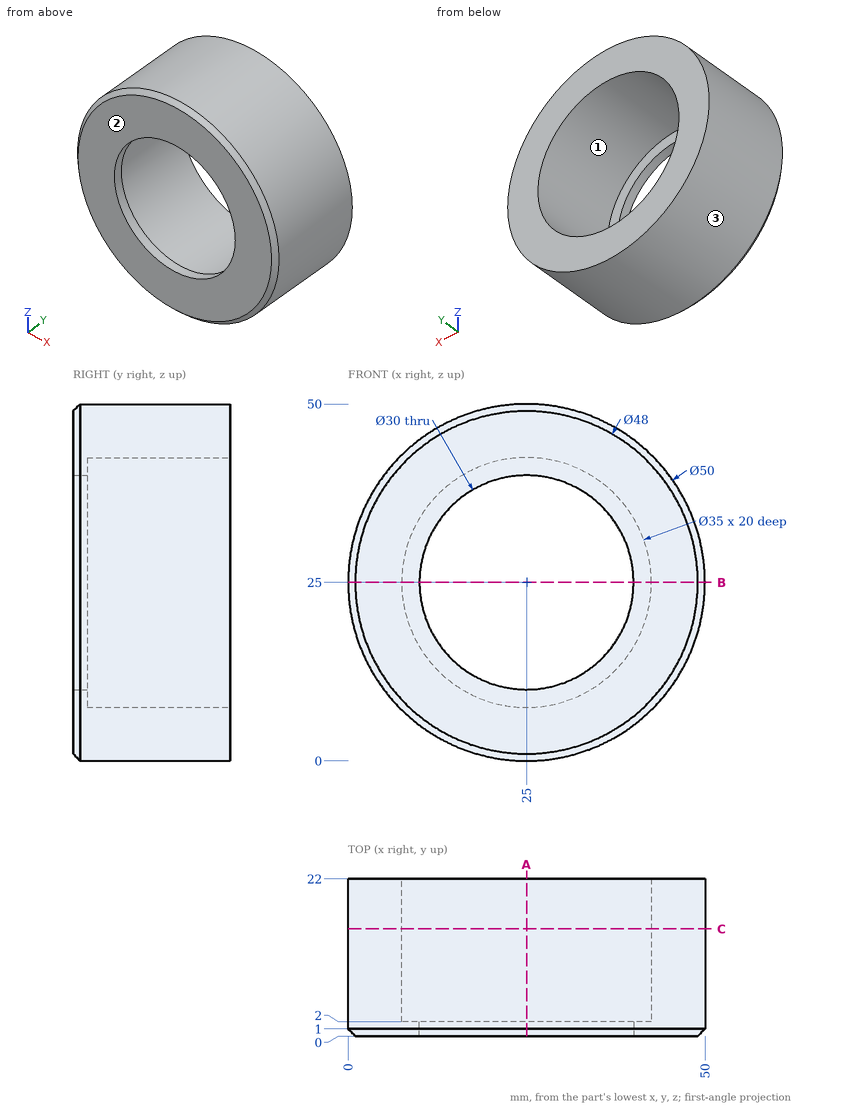
Study the drawing (mm; zero at the part's minimum x, y, z) and answer. Round coordinates to 2 decimals unless told otherwise and drop trailing zeros. Loops run counter-clockwise (first coordinate to the right, second up) from the corner with the lowest first, then second, coordinate; pieces in that order, holes last.
Q1. Find the intervals of material crossed by line 1 (X direction, y = 8.75, z = 25.5) (3 decimals); line 2 (Z direction, x = 25, y = 9.75); line 3 (Z direction, x = 25, y = 1.1), in increasing order.
Q2. Section B-B, the plane z = 25 is taken. Determine the outline of the cut face in (x, y).
Q3. Section A-A, the plane x = 25 is taken. Determine the outline of the cut face in (y, z).
Q4. Section C-C, the plane y = 15 is taken. Determine the outline of the cut face in (x, z).
Q5. For a pull along Z with two mould halves and no side action, classify the marked faces 1, 2 and 3 as released by +Z, released by -Z, zero draft, split by the parting line, or undercut.
Q6. Given pin 1 Ø5 at (x, y) = (28, 19.5) entering from +Z (3 decimals); pin 2 Ø2 at (y, z) = (17.5, 20) entering from -X; pin 3 Ø2 at (x, y) = (30.5, 11.5) entering from -Z, each flat-ended and moving along its own axis, determine where each tip first touches the part or whether it passes through.
Completed:
1. line 1: x = 0.005 to 7.507, 42.493 to 49.995
1. line 2: z = 0 to 7.5, 42.5 to 50
1. line 3: z = 0 to 10, 40 to 50
2. outline: (0, 1) - (1, 0) - (10, 0) - (10, 2) - (7.5, 2) - (7.5, 22) - (0, 22) - close; (40, 0) - (49, 0) - (50, 1) - (50, 22) - (42.5, 22) - (42.5, 2) - (40, 2) - close
3. outline: (0, 1) - (1, 0) - (22, 0) - (22, 7.5) - (2, 7.5) - (2, 10) - (0, 10) - close; (0, 40) - (2, 40) - (2, 42.5) - (22, 42.5) - (22, 50) - (1, 50) - (0, 49) - close
4. outline: circle Ø50 at (25, 25); hole circle Ø35 at (25, 25)
5. face 1: undercut
5. face 2: zero draft
5. face 3: split by the parting line
6. pin 1: stops at z = 49.995
6. pin 2: stops at x = 0.32
6. pin 3: stops at z = 0.41
